from build123d import *

# Parameters (mm, degrees)
SKETCH1_W           = 42
SKETCH1_H           = 43
BOSS_EXTRUDE1_DEPTH = 8
SKETCH2_R           = 2.1
CUT_EXTRUDE1_DEPTH  = 10
SKETCH3_R           = 2.1
CUT_EXTRUDE2_DEPTH  = 10


with BuildPart() as part:
    # Sketch1 → Boss-Extrude1 (new body)
    with BuildSketch(Plane.XY):
        with Locations((21, 21.5)):
            Rectangle(SKETCH1_W, SKETCH1_H)
    extrude(amount=BOSS_EXTRUDE1_DEPTH)

    # Sketch2 → Cut-Extrude1 (cut)
    with BuildSketch(Plane.XZ):
        with Locations((37, 4)):
            Circle(SKETCH2_R)
        with Locations((7, 4)):
            Circle(SKETCH2_R)
    extrude(amount=-CUT_EXTRUDE1_DEPTH, mode=Mode.SUBTRACT)

    # Sketch3 → Cut-Extrude2 (cut)
    with BuildSketch(Plane(origin=(0, 43, 0), x_dir=(1, 0, 0), z_dir=(0, 1, 0))):
        with Locations((37, -4)):
            Circle(SKETCH3_R)
        with Locations((7, -4)):
            Circle(SKETCH3_R)
    extrude(amount=-CUT_EXTRUDE2_DEPTH, mode=Mode.SUBTRACT)


solid = part.part
Here's how the part is built. I have some questions about the finished solid (model axes, mm). A direction names the side the tool comes from. Coordinates: 2 decimals unless noted, no trailing zeros. Order: outer loops, then holes, each group sorted by start corner. A loop starts at its lowest first (then second) coordinate and runs counter-clockwise, first axis right, second up.
Item 1: I need wall thicknesses on line 1 (Z direction, x = 37, y = 4.25); line 2 (X direction, y = 5.5, z = 3.5); line 3 (Y direction, x = 7.5, z = 6). Which ranges of each line are inside material? Lowest first, please.
Result sheet:
line 1: z = 0 to 1.9, 6.1 to 8
line 2: x = 0 to 4.96, 9.04 to 34.96, 39.04 to 42
line 3: y = 10 to 33
Item 2: If we section it at C-C on y = 6: List the corners of the cut face in (x, z) for me.
Result sheet:
outline: (0, 0) - (42, 0) - (42, 8) - (0, 8) - close; hole circle Ø4.2 at (7, 4); hole circle Ø4.2 at (37, 4)
Item 3: If we mould it in two halves opening along X, with no side actions, what happens to faces 1 (the face through (37, 10, 4)), 2 (the face through (21, 43, 4)), 3 (the face through (0, 21, 4))? For each: +X half, -X half, draft (parallel to the pull), parting line (faces both ways), or undercut.
Result sheet:
face 1: undercut
face 2: draft
face 3: -X half
Item 4: If we section it at D-D on x = 38: List the corners of the cut face in (y, z) for me.
Result sheet:
outline: (0, 0) - (43, 0) - (43, 2.15) - (33, 2.15) - (33, 5.85) - (43, 5.85) - (43, 8) - (0, 8) - (0, 5.85) - (10, 5.85) - (10, 2.15) - (0, 2.15) - close
Item 5: For faces 4 (the face through (6.54, 38.07, 6.05)), 5 (the face through (34.9, 4.93, 4.09)), 6 (the face through (21, 22, 0)), which set-ups out of +Z, -Z, +X, -X, +Y, -Y let a thin tool reach every point of the face, with its end or its side?
Result sheet:
face 4: +Y
face 5: -Y
face 6: -Z, +X, -X, +Y, -Y
Item 6: If we section it at A-A on x = 7: List the corners of the cut face in (y, z) for me, plus the area to 3 significant figures.
Result sheet:
outline: (0, 0) - (43, 0) - (43, 1.9) - (33, 1.9) - (33, 6.1) - (43, 6.1) - (43, 8) - (0, 8) - (0, 6.1) - (10, 6.1) - (10, 1.9) - (0, 1.9) - close
area: 260 mm2
Item 7: If we section it at B-B on z = 4: List the corners of the cut face in (x, y) for me.
Result sheet:
outline: (0, 0) - (4.9, 0) - (4.9, 10) - (9.1, 10) - (9.1, 0) - (34.9, 0) - (34.9, 10) - (39.1, 10) - (39.1, 0) - (42, 0) - (42, 43) - (39.1, 43) - (39.1, 33) - (34.9, 33) - (34.9, 43) - (9.1, 43) - (9.1, 33) - (4.9, 33) - (4.9, 43) - (0, 43) - close
Item 8: For P1, Ø12, axis at x = 27.5, y = 29, coming from the -Z side; P2, Ø2, axis at x = 7.5, z = 3.5, coming from the +Y side; P3, Ø3.5, axis at x = 7, z = 4, coming from the -Y side, each with a flat end and sliding along its axis, tell me the tip position at first contact or that it passes through.
Result sheet:
P1: stops at z = 0
P2: stops at y = 33
P3: stops at y = 10
